Source: CAD feature listing. Evaluate the final solid. Frame: model axes, mm. Coordinates: 2 decimals unless noted, no trailing zeros. Order: outer loops, then holes, each group sorted by start corner. A loop starts at its lowest first (then second) coordinate and runs counter-clockwise, first axis right, second up.
```python
from build123d import *

# Parameters (mm, degrees)
BOSS_EXTRUDE1_DEPTH      = 25.4
SKETCH2_W                = 19.05
SKETCH2_H                = 19.05
CUT_EXTRUDE1_DEPTH       = 1062.13626679
CUT_EXTRUDE4_DEPTH       = 26.4
SKETCH4_R                = 2.5019
SKETCH4_R_2              = 2.4892
CUT_EXTRUDE5_DEPTH       = 26.4
SKETCH6_R                = 2.4892
CUT_EXTRUDE7_DEPTH       = 539.684978519
SKETCH7_R                = 3.175
CUT_EXTRUDE8_DEPTH       = 26.4
CUT_EXTRUDE14_DEPTH      = 3.175
SKETCH16_R               = 2.4892
CUT_EXTRUDE15_DEPTH      = 23.225
CUT_EXTRUDE15_DEPTH_BACK = 4.175
SKETCH17_R               = 2.4892
CUT_EXTRUDE16_DEPTH      = 519.943248576


with BuildPart() as part:
    # Sketch1 → Boss-Extrude1 (new body)
    with BuildSketch(Plane(origin=(0, 0, 0), x_dir=(1, 0, 0), z_dir=(0, 1, 0))):
        Polygon((-584.2, 762), (-584.2, 721.632068306), (0, 0), (0, 40.367931694), align=None)
        Polygon((0, 40.367931694), (32.680013447, 0), (0, 0), align=None)
        Polygon((-635, 824.750614635), (-584.2, 762), (-584.2, 721.632068306), (-635, 784.382682941), align=None)
    extrude(amount=BOSS_EXTRUDE1_DEPTH)

    # Sketch2 → Cut-Extrude1 (cut, through all)
    with BuildSketch(Plane(origin=(12.938283504, 0, 15.981992956), x_dir=(0, -1, 0), z_dir=(0.629212321, 0, 0.777233462))):
        with Locations((-12.7, 12.7)):
            Rectangle(SKETCH2_W, SKETCH2_H)
    extrude(amount=-CUT_EXTRUDE1_DEPTH, mode=Mode.SUBTRACT)

    # Sketch3 → Cut-Extrude4 (cut, through all)
    with BuildSketch(Plane(origin=(0, 25.4, 0), x_dir=(1, 0, 0), z_dir=(0, 1, 0))):
        Polygon((25.4, 8.992624377), (25.4, 0), (32.680013447, 0), align=None)
    extrude(amount=-CUT_EXTRUDE4_DEPTH, mode=Mode.SUBTRACT)

    # Sketch4 → Cut-Extrude5 (cut, through all)
    with BuildSketch(Plane.XZ):
        with Locations((-571.537427097, -1019.306313169)):
            Circle(SKETCH4_R)
        with Locations((-565.206140645, -1008.297007475)):
            Circle(SKETCH4_R)
        with Locations((6.35, -12.7)):
            Circle(SKETCH4_R_2)
    extrude(amount=-CUT_EXTRUDE5_DEPTH, mode=Mode.SUBTRACT)

    # Sketch6 → Cut-Extrude7 (cut, through all)
    with BuildSketch(Plane(origin=(0, 0, 0), x_dir=(0.629212321, 0, 0.777233462), z_dir=(-0.777233462, 0, 0.629212321))):
        with Locations((-12.7, 12.7)):
            Circle(SKETCH6_R)
    extrude(amount=-CUT_EXTRUDE7_DEPTH, mode=Mode.SUBTRACT)

    # Sketch7 → Cut-Extrude8 (cut, through all)
    with BuildSketch(Plane(origin=(0, 25.4, 0), x_dir=(1, 0, 0), z_dir=(0, 1, 0))):
        with Locations((-292.1, 381)):
            Circle(SKETCH7_R)
    extrude(amount=-CUT_EXTRUDE8_DEPTH, mode=Mode.SUBTRACT)

    # Sketch15 → Cut-Extrude14 (cut)
    with BuildSketch(Plane.XZ):
        Polygon((-635, -784.382682941), (-635, -824.750614635), (-584.2, -762), (-584.2, -721.632068306), align=None)
    extrude(amount=-CUT_EXTRUDE14_DEPTH, mode=Mode.SUBTRACT)

    # Sketch16 → Cut-Extrude15 (cut, two sides)
    with BuildSketch(Plane.XZ.offset(-22.225)) as cut_extrude15_sk:
        with Locations((-603.036014087, -765.083188902)):
            Circle(SKETCH16_R)
        with Locations((-619.018007044, -784.824918845)):
            Circle(SKETCH16_R)
    extrude(amount=CUT_EXTRUDE15_DEPTH, mode=Mode.SUBTRACT)
    extrude(cut_extrude15_sk.sketch, amount=-CUT_EXTRUDE15_DEPTH_BACK, mode=Mode.SUBTRACT)

    # Sketch17 → Cut-Extrude16 (cut, through all)
    with BuildSketch(Plane(origin=(19.741729943, 0, -15.981992956), x_dir=(-0.629212321, 0, -0.777233462), z_dir=(0.777233462, 0, -0.629212321))):
        with Locations((697.673599675, 12.7)):
            Circle(SKETCH17_R)
        with Locations((672.273599675, 12.7)):
            Circle(SKETCH17_R)
        with Locations((646.873599675, 12.7)):
            Circle(SKETCH17_R)
    extrude(amount=-CUT_EXTRUDE16_DEPTH, mode=Mode.SUBTRACT)


solid = part.part
```
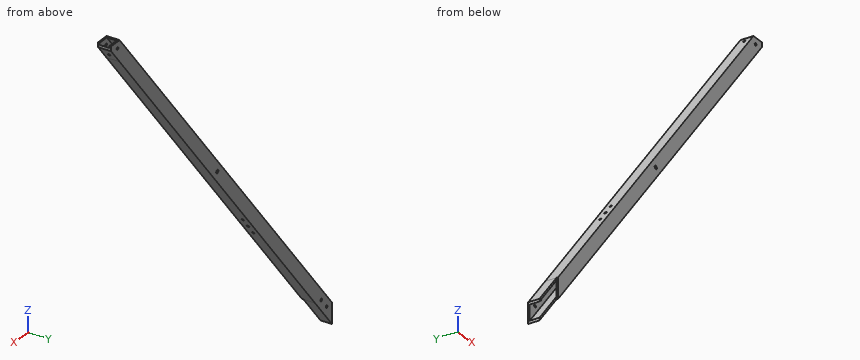
Q1. Material intervals for line 1 along Y through (x, z) = (-95.5, -142) (3 decimals); line 2 along Z through (x, y) = (-88.5, 20.25); line 3 along Z through (x, y) = (-292.1, 23.65) (3 decimals), sorted ascending.
Solutions:
line 1: y = 0 to 3.175, 22.225 to 25.4
line 2: z = -149.69 to -144.64, -114.37 to -109.32
line 3: z = -401.184 to -384.175, -377.825 to -360.816
Q2. Section query A-A on x = -139. Output: boundary loops of the cut face in (y, z) (1 decimal), plus the area to 3 significant figures.
Solutions:
outline: (0, -212.1) - (25.4, -212.1) - (25.4, -171.7) - (0, -171.7) - close; hole (3.2, -207) - (22.2, -207) - (22.2, -176.7) - (3.2, -176.7) - close
area: 449 mm2
Q3. Section query B-B on z = -486.5. Output: boundary loops of the cut face in (x, y) (3 decimals).
Solutions:
outline: (-393.848, 0) - (-361.168, 0) - (-361.168, 25.4) - (-393.848, 25.4) - close; hole (-389.763, 3.175) - (-365.253, 3.175) - (-365.253, 22.225) - (-389.763, 22.225) - close
Q4. Pin query (flat end, axial travel): P1, Ø8, axis at x = 6.35, z = -12.7, coming from the +Y side; P2, Ø3, axis at x = -552, y = 7, coming from the +Z side; P3, Ø3, axis at y = 4.5, z = -501.5, coming from the +X side; P4, Ø1, axis at x = -428.5, y = 19.5, coming from the -Z side. Return the tip coordinate at first contact, or that it passes through.
Solutions:
P1: stops at y = 25.4
P2: stops at z = -680
P3: stops at x = -372.1
P4: stops at z = -570.29
